```python
from build123d import *

# Parameters (mm, degrees)
F0_R     = 1.55
F0_R_2   = 1.25
F1_DEPTH = 1
F2_R     = 5


with BuildPart() as f1:
    # F0 (on Top) → F1 (new body)
    with BuildSketch(Plane.XY):
        with BuildLine():
            ThreePointArc((0, 23.458341), (-13.001904, 28.47242), (-19.270611, 40.918055))
            ThreePointArc((-19.270611, 40.918055), (-25.220675, 44.3861), (-26.652391, 37.649574))
            ThreePointArc((-26.652391, 37.649574), (-20.826638, 27.482582), (-19.764921, 15.812969))
            ThreePointArc((-19.764921, 15.812969), (-19.018125, 12.699808), (-16.405741, 10.849155))
            Line((-16.405741, 10.849155), (-16.405741, 0))
            Line((-16.405741, 0), (-9.353283, 0))
            Line((-9.353283, 0), (-9.353283, 9.622366))
            Line((-9.353283, 9.622366), (0, 9.622366))
            Line((0, 9.622366), (0, 23.458341))
        make_face()
        with Locations((-15.249896, 15.249896)):
            Circle(F0_R, mode=Mode.SUBTRACT)
        with Locations((-23.5, 40.5)):
            Circle(F0_R_2, mode=Mode.SUBTRACT)
    extrude(amount=F1_DEPTH)

    # F2
    f2_edges = [f1.edges().sort_by_distance(p)[0] for p in [
        (-9.353283, 9.622366, 0.5),
        (-16.405741, 10.849155, 0.5),
    ]]
    fillet(f2_edges, radius=F2_R)

    # F3: F1 across face


with BuildPart() as f1_1:
    add(f1.part)
    add(f1.part.mirror(Plane(origin=(-12.879512, 0, 0.5), x_dir=(1, 0, 0), z_dir=(0, -1, 0))))

    # F4: F1 across face


with BuildPart() as f1_2:
    add(f1_1.part)
    add(f1_1.part.mirror(Plane(origin=(0, 16.540354, 0.5), x_dir=(0, 1, 0), z_dir=(1, 0, 0))))


solid = f1_2.part
```
Geometry check sheet. Reference: the model listing, model coordinates, mm. A direction names the side the tool comes from. Round coordinates to 2 decimals unless told otherwise and drop trailing zeros. Order: outer loops, then holes, each group sorted by start corner. A loop starts at its lowest first (then second) coordinate and runs counter-clockwise, first axis right, second up. Notation, with made-up numbers: (79, -1.75) - (135, -1.75) arc R28 cw to (135, 25.25) - close; hole circle Ø2 at (56.5, -25.5). An arc over 180 degrees is marked (long way). Use a Markdown table: item, result. Add a question column.
1) Section check A-A (y = 2). Record the cut outline in (x, z), then the cut area to 3 significant figures.
2) Section check D-D (x = 23.5). Record the cut outline in (y, z), then the cut area to 3 significant figures.
3) Section check B-B (x = 5.5). Record the cut outline in (y, z).
4) Set-up check for faces 1 (the cylindrical face through (-7.85, -8.197, 0.507)), 2 (the cylindrical face through (16.885, -10.084, 0.507)), 3 (the cylindrical face through (-16.885, 10.084, 0.507)): record each of +Z, -Z, +X, -X, +Y, -Y from which the full face is reachable in a straight line by a thin tool's end or side.
5) Section check C-C (x = -15.5). Record the cut outline in (y, z), then the cut area to 3 significant figures.
6) Thickness scan on line 1 along Y through (x, z) = (0.5, 0.2); line 2 along Y through (x, z) = (15, 0.65); line 3 along X through (y, z) = (-4.5, 0.1). Record the ranges inside material, lowest first.
7) Gauge pin test, flat end, axial feed: P1, Ø0.5, axis at y = 0, z = 0.5, coming from the +X side. Record the tip position at first contact, or that the pin passes through.
Established:
| question | item | result |
|---|---|---|
| 1 | outline | (-16.41, 0) - (-9.35, 0) - (-9.35, 1) - (-16.41, 1) - close; (9.35, 0) - (16.41, 0) - (16.41, 1) - (9.35, 1) - close |
| 1 | area | 14.1 mm2 |
| 2 | outline | (-44.75, 0) - (-41.75, 0) - (-41.75, 1) - (-44.75, 1) - close; (-39.25, 0) - (-33.41, 0) - (-33.41, 1) - (-39.25, 1) - close; (33.41, 0) - (39.25, 0) - (39.25, 1) - (33.41, 1) - close; (41.75, 0) - (44.75, 0) - (44.75, 1) - (41.75, 1) - close |
| 2 | area | 17.7 mm2 |
| 3 | outline | (-24.26, 0) - (-9.49, 0) - (-9.49, 1) - (-24.26, 1) - close; (9.49, 0) - (24.26, 0) - (24.26, 1) - (9.49, 1) - close |
| 4 | face 1 | +Z, -Z |
| 4 | face 2 | +Z, -Z, +X |
| 4 | face 3 | +Z, -Z, -X |
| 5 | outline | (-31.22, 0) - (-16.78, 0) - (-16.78, 1) - (-31.22, 1) - close; (-13.72, 0) - (13.72, 0) - (13.72, 1) - (-13.72, 1) - close; (16.78, 0) - (31.22, 0) - (31.22, 1) - (16.78, 1) - close |
| 5 | area | 56.3 mm2 |
| 6 | line 1 | -23.46 to -9.62, 9.62 to 23.46 |
| 6 | line 2 | -30.58 to -16.78, -13.72 to 13.72, 16.78 to 30.58 |
| 6 | line 3 | -16.41 to -9.35, 9.35 to 16.41 |
| 7 | P1 | x = 16.41 |
